The figure shows three views and two pictorial views of one solid part (mm, origin at its lowest corner). Answer the questions. A direction names the side the tool comes from. Round coordinates to 2 decimals unless told otherwise and drop trailing zeros. Write each loop counter-clockwise with the first axis right and the second up, starting at its lowest first coordinate (ties: lowest second). Pieces come first, ordered by that corner, then holes. Notation, with made-up numbers: (-17, 1.25) -> (3, 1.25) arc R22 cw to (3, 11.25) -> close; hole circle Ø2 at (54.5, 5.5). An arc over 180 degrees is marked (long way). One line per item, written item: value.
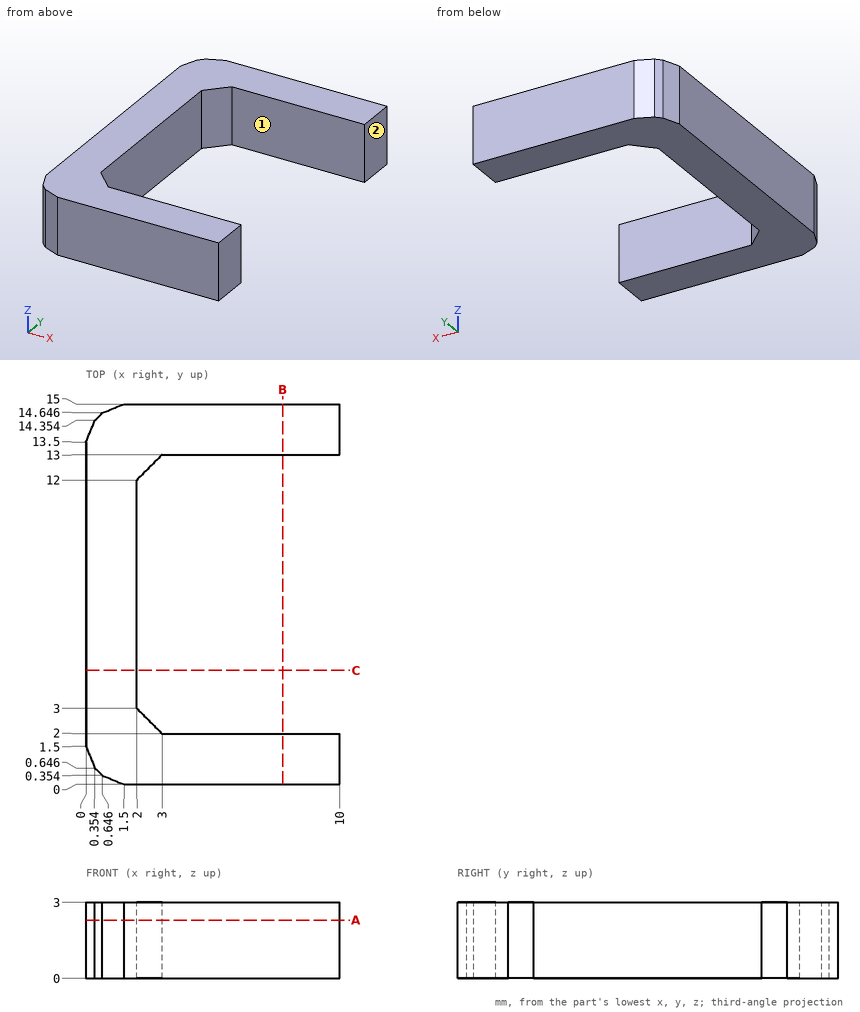
(1) Flat-ended cylindrical pins translate along their axes: pin 1 Ø1.5 at (y, z) = (5.5, 2) entering from +X; pin 2 Ø1 at (y, z) = (4.5, 1.5) entering from -X. Find the tip coordinate at first contact, or state that the pin passes through.
Reported:
pin 1: stops at x = 2
pin 2: stops at x = 0
(2) Find section B-B on x = 7.75. Give the vertices of the cut face in (y, z), plus the area to 3 significant figures.
Reported:
outline: (0, 0) -> (2, 0) -> (2, 3) -> (0, 3) -> close; (13, 0) -> (15, 0) -> (15, 3) -> (13, 3) -> close
area: 12.0 mm2
(3) Find section A-A on z = 2.3. Give the vertices of the cut face in (x, y).
Reported:
outline: (0, 1.5) -> (0.35, 0.65) -> (0.65, 0.35) -> (1.5, 0) -> (10, 0) -> (10, 2) -> (3, 2) -> (2, 3) -> (2, 12) -> (3, 13) -> (10, 13) -> (10, 15) -> (1.5, 15) -> (0.65, 14.65) -> (0.35, 14.35) -> (0, 13.5) -> close
(4) Consider probe 1 along Y at (x, z) = (7.25, 0.7); probe 2 along X at (y, z) = (4, 2.55); probe 3 along Y at (x, z) = (2.75, 0.75). Determine where each line is inside the solid, lowest interval first.
Reported:
probe 1: y = 0 to 2, 13 to 15
probe 2: x = 0 to 2
probe 3: y = 0 to 2.25, 12.75 to 15
(5) A tool of negligible diameter and unlimited length cuts with its end or side. For the marked faces 1 and 2, from which of +Z, -Z, +X, -X, +Y, -Y can it reach the whole face along a straight path? Write none if from no direction.
Reported:
face 1: +Z, -Z, +X
face 2: +Z, -Z, +X, +Y, -Y
(6) Find section C-C on y = 4.5. Give the vertices of the cut face in (x, z).
Reported:
outline: (0, 0) -> (2, 0) -> (2, 3) -> (0, 3) -> close
